Autodesk Inventor part; units mm, degrees
ref_plane "YZ Plane" through (0, 0, 0) normal (1, 0, 0) x (0, 1, 0)
ref_plane "XZ Plane" through (0, 0, 0) normal (0, 1, 0) x (-1, 0, 0)
ref_plane "XY Plane" through (0, 0, 0) normal (0, 0, 1) x (1, 0, 0)
sketch "Sketch1" plane through (0, 0, 0) normal (0, 0, 1) x (1, 0, 0)
  arc A0 (187.325, 0) -> (0, 187.325) centre (0, 0) ccw
  arc A1 (136.525, 0) -> (0, 136.525) centre (0, 0) ccw
  line L0 (0, 136.525) -> (0, 187.325)
  line L1 (136.525, 0) -> (187.325, 0)
  point P0 (161.925, 0)
  point P1 (0, 161.925)
  dimension "d2" = 187.325
  dimension "d3" = 136.525
extrude "Extrusion1" add sketch "Sketch1" along normal blind 0.4
sketch "Sketch3" plane through (0, 0, 0.4) normal (0, 0, 1) x (1, 0, 0)
  line L0 (178.117, 32.1925) -> (176.8782, 38.4205)
  arc A0 (178.117, 32.1925) -> (181.231, 32.8119) centre (179.674, 32.5022) ccw
  line L1 (179.9922, 39.0399) -> (181.231, 32.8119)
  arc A1 (179.9922, 39.0399) -> (176.8782, 38.4205) centre (178.4352, 38.7302) ccw
  line L2 (130.2137, 125.7236) -> (125.7236, 130.2137)
  arc A2 (130.2137, 125.7236) -> (132.4588, 127.9686) centre (131.3362, 126.8461) ccw
  arc A3 (127.9686, 132.4588) -> (125.7236, 130.2137) centre (126.8461, 131.3362) ccw
  line L3 (127.9686, 132.4588) -> (132.4588, 127.9686)
  line L4 (38.4205, 176.8782) -> (32.1925, 178.117)
  arc A4 (38.4205, 176.8782) -> (39.0399, 179.9922) centre (38.7302, 178.4352) ccw
  line L5 (32.8119, 181.231) -> (39.0399, 179.9922)
  arc A5 (32.8119, 181.231) -> (32.1925, 178.117) centre (32.5022, 179.674) ccw
  arc A6 (0, 161.925) -> (0, 151.3184) centre (-0.5713, 156.6217) ccw
  circle A7 centre (-0.5713, 156.6217) radius 5.334
  point P0 (0, 0)
  point P1 (0, 161.925)
extrude "Extrusion2" cut sketch "Sketch3" against normal through all
properties part number "3DPRINT,CABLE,TRAY" material "ABS Plastic"
Check sheet for the modelled part. Datum: model origin and axes. Units: mm. A direction names the side the tool comes from. Coordinates: 2 decimals unless noted, no trailing zeros. Write each loop counter-clockwise with the first axis right and the second up, starting at its lowest first coordinate (ties: lowest second). Pieces come first, ordered by that corner, then holes. Notation, with made-up numbers: M -29.5,44 L 26.5,44 A35 ccw 26.5,77 Z; hole C 32.5,27 d3. An arc over 180 degrees is marked long. Answer as CSV lines item,"result".
Q1. Cross-section at B-B (y = 96.5). Record the boundary of the cut face in (x, z), then the cut area to 3 significant figures.
Check result:
outline,"M 96.58,0 L 160.56,0 L 160.56,0.4 L 96.58,0.4 Z"
area,"25.6 mm^2"
Q2. Mould release check, pull along Y, two halves, no side actions. Record for faces 1 (the face through (95.47, 97.593, 0.197)), 2 (the face through (92, 116, 0.4)), 3 (the face through (4.76, 156.51, 0.2)): released by +Y, released by -Y, zero draft, split by the parting line, or undercut.
Check result:
face 1,"released by -Y"
face 2,"zero draft"
face 3,"undercut"
Q3. Material ranges on probe 1 along X at (y, z) = (37.5, 0.1); probe 2 along X at (y, z) = (35, 0.25); probe 3 along X at (y, z) = (74, 0.2), recorded low to high. Write a range as from..to.
Check result:
probe 1,"131.27..177.06, 180.3..183.53"
probe 2,"131.96..177.56, 180.8..184.03"
probe 3,"114.73..172.09"
Q4. Cross-section at A-A (z = 0.15). Count the separate pieces of the cut face and the enclosed holes in it, then the cut area to 3 significant figures.
Check result:
separate pieces,"1"
enclosed holes,"3"
area,"12,800 mm^2"
Q5. Cross-section at C-C (x = 11.5). Record the boundary of the cut face in (y, z).
Check result:
outline,"M 136.04,0 L 186.97,0 L 186.97,0.4 L 136.04,0.4 Z"
Q6. Go/stop test with a flat-tipped pin: pin 1 (1 mm diameter, centred on x = 160, y = 98.5, fed in from -Z). Record where the tip stops, or that it passes through.
Check result:
pin 1,"through"
Q7. Set-up check for faces 4 (the face through (92, 116, 0)), 5 (the face through (128, 127.94, 0.2)): record each of +Z, -Z, +X, -X, +Y, -Y from which the full face is reachable in a straight line by a thin tool's end or side.
Check result:
face 4,"-Z, +X, -X, +Y, -Y"
face 5,"+Z, -Z"
